```python
from build123d import *

# Parameters (mm, degrees)
SKETCH1_W           = 6
SKETCH1_H           = 6
BOSS_EXTRUDE2_DEPTH = 6


with BuildPart() as part:
    # Sketch1 → Boss-Extrude2 (new body)
    with BuildSketch(Plane(origin=(0, 0, 0), x_dir=(1, 0, 0), z_dir=(0, 1, 0))):
        Polygon((0, 0), (-3, 0), (-3, 6), (-9, 6), (-9, 0), (-21, 0), (-21, 6), (-27, 6), (-27, 0), (-30, 0), (-30, -100), (-27, -100), (-27, -106), (-21, -106), (-21, -100), (-9, -100), (-9, -106), (-3, -106), (-3, -100), (0, -100), align=None)
        with Locations((-15, -57)):
            Rectangle(SKETCH1_W, SKETCH1_H, mode=Mode.SUBTRACT)
        with Locations((-6, -57)):
            Rectangle(SKETCH1_W, SKETCH1_H, mode=Mode.SUBTRACT)
        with Locations((-24, -57)):
            Rectangle(SKETCH1_W, SKETCH1_H, mode=Mode.SUBTRACT)
        with Locations((-15, -13)):
            Rectangle(SKETCH1_W, SKETCH1_H, mode=Mode.SUBTRACT)
        with Locations((-6, -13)):
            Rectangle(SKETCH1_W, SKETCH1_H, mode=Mode.SUBTRACT)
        with Locations((-24, -13)):
            Rectangle(SKETCH1_W, SKETCH1_H, mode=Mode.SUBTRACT)
    extrude(amount=BOSS_EXTRUDE2_DEPTH)


solid = part.part
```
Can you work these out from the model? Positions are in its coordinate system, mm. A direction names the side the tool comes from. Round coordinates to 2 decimals unless told otherwise and drop trailing zeros. Loops run counter-clockwise (first coordinate to the right, second up) from the corner with the lowest first, then second, coordinate; pieces in that order, holes last. Notation, with made-up numbers: M 63.5,-37 L 83.5,-37 A13 ccw 83.5,-26 Z; hole C 44.25,35 d9. An arc over 180 degrees is marked long. Write item = value, one per line. Start each with the question number.
(1) Which directions (+Z, -Z, +X, -X, +Y, -Y) give clear straight access to the entire face, cutting with the end or side of a thin tool? Please do faces 5 (the face through (-15, 3, 60)), 6 (the face through (-3, 3, -3)), 7 (the face through (-9, 3, 103)).
(2) Suppose I cut it at B-B on x = -15.75. Write out the boundary of the cut face in (y, z).
(3) Suppose I cut it at C-C on y = 4.5. Give the number of separate pieces and of enclosed holes in the cut face, plus the area to 3 significant figures.
(4) I need wall thicknesses on line 1 along Z through (x, y) = (-7.25, 3.75); line 2 along Z through (x, y) = (-14.25, 2.9); line 3 along Z through (x, y) = (-9.5, 0.4). Which ranges of each line are inside material? Lowest first, please.
(5) Suppose I cut it at D-D on x = -28. Write out the boundary of the cut face in (y, z).
(6) Suppose I cut it at A-A on z = 56.5. Write out the boundary of the cut face in (x, y).
(7) I'm going to push flat-ended pins straight in: P1, Ø1.8, axis at y = 4, z = 104.5, coming from the -X side; P2, Ø1.5, axis at x = -25.5, z = 70.5, coming from the -Y side; P3, Ø1, axis at x = -18.5, y = 4.5, coming from the +Z side. Where does each tip first touch, or does it pass through?
(8) If we mould it in two halves opening along Z, with no side actions, what happens to faces 1 (the face through (-24, 3, 106)), 2 (the face through (-1, 3, 0)), 3 (the face through (-15, 3, 10)), 4 (the face through (-21, 3, -3))? For each: released by +Z, released by -Z, zero draft, split by the parting line, or undercut.
Answer block:
q1.face_5 = +Y, -Y
q1.face_6 = -Z, +X, +Y, -Y
q1.face_7 = +Z, +Y, -Y
q2.outline = M 0,0 L 6,0 L 6,10 L 0,10 Z; M 0,16 L 6,16 L 6,54 L 0,54 Z; M 0,60 L 6,60 L 6,100 L 0,100 Z
q3.separate_pieces = 1
q3.enclosed_holes = 6
q3.area = 2,930 mm²
q4.line_1 = -6 to 10, 16 to 54, 60 to 106
q4.line_2 = 0 to 10, 16 to 54, 60 to 100
q4.line_3 = 0 to 100
q5.outline = M 0,0 L 6,0 L 6,100 L 0,100 Z
q6.outline = M -30,0 L -27,0 L -27,6 L -30,6 Z; M -21,0 L -18,0 L -18,6 L -21,6 Z; M -12,0 L -9,0 L -9,6 L -12,6 Z; M -3,0 L 0,0 L 0,6 L -3,6 Z
q7.P1 = -27
q7.P2 = 0
q7.P3 = 100
q8.face_1 = released by +Z
q8.face_2 = released by -Z
q8.face_3 = undercut
q8.face_4 = zero draft
